Verification items for the finished model (mm, model axes). Round coordinates to 2 decimals unless told otherwise and drop trailing zeros. Loops run counter-clockwise (first coordinate to the right, second up) from the corner with the lowest first, then second, coordinate; pieces in that order, holes last. Notation, with made-up numbers: (64.5, -1.75) -> (111.5, -1.75) arc R10 cw to (111.5, 5.25) -> close; hole circle Ø6 at (66, 58). An arc over 180 degrees is marked (long way). Use a Markdown table: item, result. Add a question column.
```python
from build123d import *

# Parameters (mm, degrees)
F2_R     = 0.75
F3_DEPTH = 3
F4_SIZE  = 0.1


with BuildPart() as f1:
    # F0 (on Front) → F1 (revolve)
    with BuildSketch(Plane.XZ):
        with BuildLine():
            Line((-1.5, 0), (0, 0))
            Line((0, 0), (1.5, 0))
            Line((1.5, 0), (1.5, 5))
            Line((1.5, 5), (0.5, 5))
            Line((0.5, 5), (0.5, 4.7))
            ThreePointArc((0.5, 4.7), (0, 4.2), (-0.5, 4.7))
            Line((-0.5, 4.7), (-0.5, 5))
            Line((-0.5, 5), (-1.5, 5))
            Line((-1.5, 5), (-1.5, 0))
        make_face()
    revolve(axis=Axis((-0.75, 0, 0), (-1, 0, 0)))

    # F2 (on face) → F3 (cut, through all)
    with BuildSketch(Plane.YZ.offset(1.5)):
        Circle(F2_R)
    extrude(amount=-F3_DEPTH, mode=Mode.SUBTRACT)

    # F4
    f4_edges = [f1.edges().sort_by_distance(p)[0] for p in [
        (0.5, 0, -5),
        (-0.5, 0, -5),
    ]]
    chamfer(f4_edges, length=F4_SIZE)


solid = f1.part
```
1) Sectioned sample at C-C on x = 0.3. Enter the section's corners in (y, z).
2) Thickness scan on line 1 (X direction, y = -0.5, z = 4.75); line 2 (Z direction, x = -1.1, y = -0.5); line 3 (Y direction, x = -0.55, z = -0.5). Record the ranges inside material, lowest first.
3) Release check for a two-part mould opening along Z. For faces 1 (the face through (0.02, -0.75, 0.03)), 2 (the face through (-1.06, -4.88, -1.08)), 3 (the face through (1.5, 0, -1)) record: released by +Z, released by -Z, zero draft, split by the parting line, or undercut.
4) Sectioned sample at A-A on y = 0. Enter the section's corners in (x, z).
5) Sectioned sample at D-D on x = -0.95. Enter the section's corners in (y, z), then the cut area to 3 significant figures.
Geometry results:
| question | item | result |
|---|---|---|
| 1 | outline | circle Ø8.6 at (0, 0); hole circle Ø1.5 at (0, 0) |
| 2 | line 1 | -1.5 to -0.5, 0.5 to 1.5 |
| 2 | line 2 | -4.97 to -0.56, 0.56 to 4.97 |
| 2 | line 3 | -4.92 to -0.56, 0.56 to 4.92 |
| 3 | face 1 | undercut |
| 3 | face 2 | split by the parting line |
| 3 | face 3 | zero draft |
| 4 | outline | (-1.5, -5) -> (-0.6, -5) -> (-0.5, -4.9) -> (-0.5, -4.7) arc R0.5 cw to (0.5, -4.7) -> (0.5, -4.9) -> (0.6, -5) -> (1.5, -5) -> (1.5, -0.75) -> (-1.5, -0.75) -> close; (-1.5, 0.75) -> (1.5, 0.75) -> (1.5, 5) -> (0.6, 5) -> (0.5, 4.9) -> (0.5, 4.7) arc R0.5 cw to (-0.5, 4.7) -> (-0.5, 4.9) -> (-0.6, 5) -> (-1.5, 5) -> close |
| 5 | outline | circle Ø10 at (0, 0); hole circle Ø1.5 at (0, 0) |
| 5 | area | 76.8 mm^2 |
